Build history of the part. All positions in model axes, mm. Face numbers are marked on the shaded views. A direction names the side the tool comes from. Give positions to 0.01 mm unless a question says otherwise; leave off trailing zeros. Loops run counter-clockwise (first coordinate to the right, second up) from the corner with the lowest first, then second, coordinate; pieces in that order, holes last. Notation, with made-up numbers: (69.25, 10) -> (83.25, 10) arc R28 cw to (83.25, 40) -> close; hole circle Ø3 at (57.25, -32.75). An arc over 180 degrees is marked (long way). One line per question, with ' | ' between items. Start each with the question number.
(1) Slice it at A-A, the plane x = 13. Write the cut outline in (y, z), then the cut area to 3 significant figures.
(2) Drill centre lines: L1, parallel to Z at x = 13, y = 27.5; L2, parallel to Z at x = 1.6, y = 12.5; L3, parallel to Z at x = 1.9, y = 6.5. Where is each one in solid material? Low to high. Write a range as from..to.
(3) 3-axis set-ups, long thin cutter, end or side, ignore diameter. For the marked faces 4 and 5: which of +Z, -Z, +X, -X, +Y, -Y reach the whole face in a straight line?
(4) Slice it at B-B, the plane z = 0. Write the cut outline in (x, y).
(5) Mould opens along Y. For the marked faces 1, 2 and 3 say: pulls with the +Y half, pulls with the -Y half, needs draft (parallel to the pull), parting line crosses it, or undercut.
(6) Slice it at D-D, the plane x = 17.5. Write the cut outline in (y, z).
(7) Slice it at C-C, the plane y = 12.5. Write the cut outline in (x, z).
(8) Flat gauge pins, fed straight in: pin 1 Ø2.5 at (y, z) = (1, -1) entering from +X; pin 2 Ø8.5 at (x, z) = (15.5, 2) entering from -Y; pin 3 Ø3.5 at (y, z) = (6.5, 0) entering from +X. Where does each tip first touch, or does it go through?
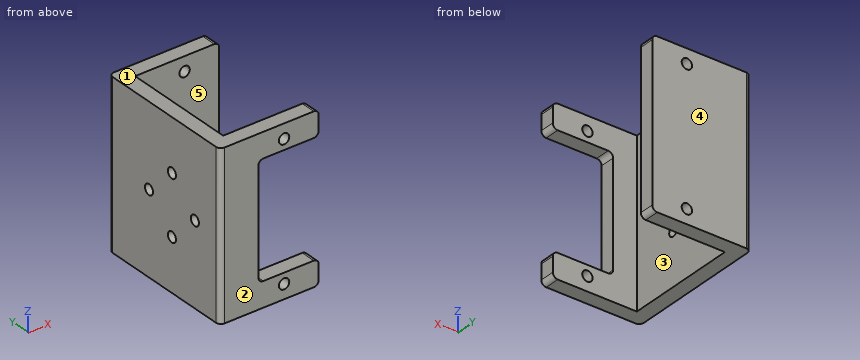
```python
from build123d import *

# Parameters (mm, degrees)
PAD_DEPTH       = 16.5
SKETCH001_R     = 1.05
POCKET_DEPTH    = 33
SKETCH002_W     = 12.2
SKETCH002_H     = 23
POCKET001_DEPTH = 5
SKETCH003_R     = 1.05
POCKET002_DEPTH = 5
FILLET_R        = 1


with BuildPart() as part:
    # Sketch → Pad (new body, symmetric)
    with BuildSketch(Plane.XY):
        Polygon((0, 0), (0, 29), (20, 29), (20, 26), (3, 26), (3, 3), (20, 3), (20, 0), align=None)
    extrude(amount=PAD_DEPTH, both=True)

    # Sketch001 → Pocket (cut)
    with BuildSketch(Plane.XZ):
        with Locations((13, 13.6)):
            Circle(SKETCH001_R)
        with Locations((13, -13.6)):
            Circle(SKETCH001_R)
    extrude(amount=-POCKET_DEPTH, mode=Mode.SUBTRACT)

    # Sketch002 (on Face2 of Pocket) → Pocket001 (cut)
    with BuildSketch(Plane.XZ):
        with Locations((13.9, 0)):
            Rectangle(SKETCH002_W, SKETCH002_H)
    extrude(amount=-POCKET001_DEPTH, mode=Mode.SUBTRACT)

    # Sketch003 (on Face1 of Pocket001) → Pocket002 (cut)
    with BuildSketch(Plane(origin=(0, 0, 0), x_dir=(0, -1, 0), z_dir=(-1, 0, 0))):
        with Locations((-12.5, 6)):
            Circle(SKETCH003_R)
        with Locations((-12.5, -6)):
            Circle(SKETCH003_R)
        with Locations((-6.5, 0)):
            Circle(SKETCH003_R)
        with Locations((-18.5, 0)):
            Circle(SKETCH003_R)
    extrude(amount=-POCKET002_DEPTH, mode=Mode.SUBTRACT)

    # Fillet
    fillet_edges = [part.edges().sort_by_distance(p)[0] for p in [
        (20, 27.5, 16.5),
        (20, 27.5, -16.5),
        (20, 1.5, 16.5),
        (20, 1.5, -16.5),
        (0, 0, 0),
        (0, 29, 0),
        (20, 1.5, -11.5),
        (20, 1.5, 11.5),
        (7.8, 1.5, -11.5),
        (7.8, 1.5, 11.5),
    ]]
    fillet(fillet_edges, radius=FILLET_R)


solid = part.part
```
Final values:
1) outline: (0, -16.5) -> (3, -16.5) -> (3, -14.65) -> (0, -14.65) -> close; (0, -12.55) -> (3, -12.55) -> (3, -11.5) -> (0, -11.5) -> close; (0, 11.5) -> (3, 11.5) -> (3, 12.55) -> (0, 12.55) -> close; (0, 14.65) -> (3, 14.65) -> (3, 16.5) -> (0, 16.5) -> close; (26, -16.5) -> (29, -16.5) -> (29, -14.65) -> (26, -14.65) -> close; (26, -12.55) -> (29, -12.55) -> (29, 12.55) -> (26, 12.55) -> close; (26, 14.65) -> (29, 14.65) -> (29, 16.5) -> (26, 16.5) -> close | area: 104 mm2
2) L1: -16.5..-14.65, -12.55..12.55, 14.65..16.5 | L2: -16.5..-7.05, -4.95..4.95, 7.05..16.5 | L3: -16.5..-1.05, 1.05..16.5
3) face 4: +Z, -Z, +X, -X, +Y | face 5: +Z, -Z, +X
4) outline: (0, 1) arc R1 ccw to (1, 0) -> (7.8, 0) -> (7.8, 3) -> (3, 3) -> (3, 5.45) -> (0, 5.45) -> close; (0, 7.55) -> (3, 7.55) -> (3, 17.45) -> (0, 17.45) -> close; (0, 19.55) -> (3, 19.55) -> (3, 26) -> (20, 26) -> (20, 29) -> (1, 29) arc R1 ccw to (0, 28) -> close
5) face 1: needs draft | face 2: pulls with the -Y half | face 3: undercut
6) outline: (0, -16.5) -> (3, -16.5) -> (3, -11.5) -> (0, -11.5) -> close; (0, 11.5) -> (3, 11.5) -> (3, 16.5) -> (0, 16.5) -> close; (26, -16.5) -> (29, -16.5) -> (29, 16.5) -> (26, 16.5) -> close
7) outline: (0, -16.5) -> (3, -16.5) -> (3, -7.05) -> (0, -7.05) -> close; (0, -4.95) -> (3, -4.95) -> (3, 4.95) -> (0, 4.95) -> close; (0, 7.05) -> (3, 7.05) -> (3, 16.5) -> (0, 16.5) -> close
8) pin 1: x = 7.8 | pin 2: y = 26 | pin 3: x = 3
